Input: part model. Units: mm. Frame: model coordinates. Coordinates: 2 decimals unless noted, no trailing zeros. Order: outer loops, then holes, each group sorted by start corner. A loop starts at its lowest first (then second) coordinate and runs counter-clockwise, first axis right, second up. Notation, with made-up numbers: M 41,70 L 49,70 A25 ccw 49,108 Z; hole C 29.25,88.5 d11. An arc over 180 degrees is marked long. Answer in a Markdown table with one row per item.
from build123d import *

# Parameters (mm, degrees)
BOSS_EXTRUDE1_DEPTH     = 2
CUT_EXTRUDE1_DEPTH      = 203.119002293
CUT_EXTRUDE1_DEPTH_BACK = 203.119002293
SKETCH2_R               = 80
CUT_EXTRUDE2_DEPTH      = 203.119002293
CUT_EXTRUDE2_DEPTH_BACK = 203.119002293


with BuildPart() as part:
    # Sketch1 → Boss-Extrude1 (new body)
    with BuildSketch(Plane.XY):
        with BuildLine():
            Line((0, 0), (7.064623984, 142.825386707))
            ThreePointArc((7.064623984, 142.825386707), (143, 0.000219219), (7.065061887, -142.825365046))
            Line((7.065061887, -142.825365046), (0, 0))
        make_face()
    extrude(amount=BOSS_EXTRUDE1_DEPTH)

    # Sketch2 → Cut-Extrude1 (cut, two sides: drawn at the far end of the back side and taken through both)
    with BuildSketch(Plane(origin=(0, 0, 0), x_dir=(-1, 0, 0), z_dir=(0, 0, -1)).offset(-CUT_EXTRUDE1_DEPTH_BACK)):
        Circle(SKETCH2_R)
    extrude(amount=CUT_EXTRUDE1_DEPTH + CUT_EXTRUDE1_DEPTH_BACK, mode=Mode.SUBTRACT)

    # Sketch3 → Cut-Extrude2 (cut, two sides: drawn at the far end of the back side and taken through both)
    with BuildSketch(Plane(origin=(0, 0, 0), x_dir=(1, 0, 0), z_dir=(0, 1, 0)).offset(-CUT_EXTRUDE2_DEPTH_BACK)):
        Polygon((3.952237194, -2), (13.952237194, 0), (3.952237194, 0), align=None)
    extrude(amount=CUT_EXTRUDE2_DEPTH + CUT_EXTRUDE2_DEPTH_BACK, mode=Mode.SUBTRACT)

    # Sketch5 → Cut-Revolve1 (revolve, cut)
    with BuildSketch(Plane(origin=(0, 0, 0), x_dir=(1, 0, 0), z_dir=(0, 1, 0))):
        Polygon((80, -2), (90, 0), (80, 0), align=None)
    revolve(axis=Axis((0, 0, 0), (0, 0, -1)), mode=Mode.SUBTRACT)


solid = part.part
1) Material intervals for probe 1 along Y at (x, z) = (131.5, 0.75); probe 2 along Y at (x, z) = (102, 1.5); probe 3 along X at (y, z) = (-94.5, 1.95), sorted ascending.
Resolved:
| item | result |
|---|---|
| probe 1 | y = -56.18 to 56.18 |
| probe 2 | y = -100.22 to 100.22 |
| probe 3 | x = 4.67 to 107.33 |
2) Cut plane C-C, the plane y = 100.5. Output: boundary loops of the cut face in (x, z), and give its area (3 significant figures).
Resolved:
| item | result |
|---|---|
| outline | M 4.97,1.8 L 13.95,0 L 101.73,0 L 101.73,2 L 4.97,2 Z |
| area | 185 mm2 |
3) Cut plane B-B, the plane z = 0.5. Output: boundary loops of the cut face in (x, y).
Resolved:
| item | result |
|---|---|
| outline | M 11.45,-142.54 A143 ccw 11.45,142.54 L 11.45,86.75 A87.5 cw 11.45,-86.75 Z |
4) Cut plane D-D, the plane y = -99. Output: boundary loops of the cut face in (x, z).
Resolved:
| item | result |
|---|---|
| outline | M 4.9,1.81 L 13.95,0 L 103.19,0 L 103.19,2 L 4.9,2 Z |
5) Mould query, pull axis Y, two halves, no side actions, for faces 1 (the face through (81.718, 1.741, 1.653)), 2 (the face through (142.968, 3.046, 0.986)), 3 (the face through (90, 2, 2)). Classes: +Y half, -Y half, draft (parallel to the pull), parting line (faces both ways), or undercut.
Resolved:
| item | result |
|---|---|
| face 1 | undercut |
| face 2 | parting line |
| face 3 | draft |
6) Cut plane A-A, the plane y = 0. Output: boundary loops of the cut face in (x, z), and give its area (3 significant figures).
Resolved:
| item | result |
|---|---|
| outline | M 80,2 L 90,0 L 143,0 L 143,2 Z |
| area | 116 mm2 |
